The listing builds one solid part. Answer for the finished solid, in the listing's coordinates (mm). A direction names the side the tool comes from. Round coordinates to 2 decimals unless told otherwise and drop trailing zeros. Loops run counter-clockwise (first coordinate to the right, second up) from the corner with the lowest first, then second, coordinate; pieces in that order, holes last. Notation, with made-up numbers: M 24.5,8 L 75.5,8 A20 cw 75.5,46 Z; hole C -11.75,19.25 d5. An arc over 180 degrees is marked long. Put each result on its own line as item: value. Start each with the question number.
(1) Section D-D, the plane z = 0.75 is taken. Count the separate pieces of the cut face and the enclosed holes in it, then the cut area to 3 significant figures.
(2) Which of the six approach directions +Z, -Z, +X, -X, +Y, -Y give full straight-line access (tool end or side, diameter ignored) to faces 4 (the face through (35, 15, 2)), 5 (the face through (37, -2.5, 2)), 6 (the face through (35, -15, 2)), 7 (the face through (-38, -2.5, 2)), 8 (the face through (-5.9, 0, 2))?
(3) Section A-A, the plane x = 4 is taken. Determine the outline of the cut face in (y, z).
(4) Section C-C, the plane x = -8.4 is taken. Determine the outline of the cut face in (y, z), then the cut area to 3 significant figures.
(5) Straight lines are drawn through the part: line 1 (X direction, y = 0, z = 2.15); line 2 (Y direction, x = 11.5, z = 3.95); line 3 (Y direction, x = -8.4, z = 2.6). For each, find the intervals that lie inside material, in ascending order.
(6) Section B-B, the plane y = 0 is taken. Determine the outline of the cut face in (x, z), then the cut area to 3 significant figures.
(7) Determine the mould class of faces 1 (the face through (-35, -15, 2)), 2 (the face through (-25.418, 3.685, 2.465)), 3 (the face through (37, 2.5, 2)) for opening direction X: released by +X, released by -X, zero draft, split by the parting line, or undercut.
(8) Flat-ended cylindrical pins translate along their axes: P1, Ø1.6, axis at x = 18.8, y = 0, coming from the -Z side; P2, Ø1.5, axis at y = -15.5, z = 3, coming from the -X side; P3, Ø2.5, axis at y = 15.5, z = 2.5, coming from the +X side. Find the tip coordinate at first contact, or state that the pin passes through.
```python
from build123d import *

# Parameters (mm, degrees)
ESQUISSE1_W                = 80
ESQUISSE1_H                = 35
BOSS_EXTRU_1_DEPTH         = 5
ESQUISSE3_W                = 5
ESQUISSE3_H                = 5
ENL_V_MAT_EXTRU_1_DEPTH    = 10
R_P_TITION_LIN_AIRE1_COUNT = 4
R_P_TITION_LIN_AIRE1_PITCH = 10
ESQUISSE4_W                = 5
ESQUISSE4_H                = 5
ENL_V_MAT_EXTRU_2_DEPTH    = 10
R_P_TITION_LIN_AIRE2_COUNT = 4
R_P_TITION_LIN_AIRE2_PITCH = 10
ESQUISSE6_W                = 22.2
ESQUISSE6_H                = 11.8
ENL_V_MAT_EXTRU_5_DEPTH    = 10
ESQUISSE7_R                = 1
ESQUISSE7_R_2              = 0.999214349
ENL_V_MAT_EXTRU_7_DEPTH    = 10
ESQUISSE8_R                = 4.5
ENL_V_MAT_EXTRU_8_DEPTH    = 10
ENL_V_MAT_EXTRU_9_DEPTH    = 10


with BuildPart() as part:
    # Esquisse1 → Boss.-Extru.1 (new body)
    with BuildSketch(Plane.XY):
        Rectangle(ESQUISSE1_W, ESQUISSE1_H)
    extrude(amount=BOSS_EXTRU_1_DEPTH)

    # Esquisse3 → Enlèv. mat.-Extru.1 (cut)
    with BuildSketch(Plane.XY):
        with Locations((37.5, -15)):
            Rectangle(ESQUISSE3_W, ESQUISSE3_H)
    enl_v_mat_extru_1 = extrude(amount=ENL_V_MAT_EXTRU_1_DEPTH, mode=Mode.SUBTRACT)

    # Répétition linéaire1: Enlèv. mat.-Extru.1 ×4
    with Locations(*[(0, i * R_P_TITION_LIN_AIRE1_PITCH, 0) for i in range(1, R_P_TITION_LIN_AIRE1_COUNT)]):
        add(enl_v_mat_extru_1, mode=Mode.SUBTRACT)

    # Esquisse4 → Enlèv. mat.-Extru.2 (cut)
    with BuildSketch(Plane.XY):
        with Locations((-37.5, -15)):
            Rectangle(ESQUISSE4_W, ESQUISSE4_H)
    enl_v_mat_extru_2 = extrude(amount=ENL_V_MAT_EXTRU_2_DEPTH, mode=Mode.SUBTRACT)

    # Répétition linéaire2: Enlèv. mat.-Extru.2 ×4
    with Locations(*[(0, i * R_P_TITION_LIN_AIRE2_PITCH, 0) for i in range(1, R_P_TITION_LIN_AIRE2_COUNT)]):
        add(enl_v_mat_extru_2, mode=Mode.SUBTRACT)

    # Esquisse6 → Enlèv. mat.-Extru.5 (cut)
    with BuildSketch(Plane.XY):
        with Locations((5.2, 0)):
            Rectangle(ESQUISSE6_W, ESQUISSE6_H)
    extrude(amount=ENL_V_MAT_EXTRU_5_DEPTH, mode=Mode.SUBTRACT)

    # Esquisse7 → Enlèv. mat.-Extru.7 (cut)
    with BuildSketch(Plane.XY):
        with Locations((18.8, 0)):
            Circle(ESQUISSE7_R)
        with Locations((-8.4, 0)):
            Circle(ESQUISSE7_R_2)
    extrude(amount=ENL_V_MAT_EXTRU_7_DEPTH, mode=Mode.SUBTRACT)

    # Esquisse8 → Enlèv. mat.-Extru.8 (cut)
    with BuildSketch(Plane(origin=(0, 0, 0), x_dir=(-1, 0, 0), z_dir=(0, 0, -1))):
        with Locations((28, 0)):
            Circle(ESQUISSE8_R)
    enl_v_mat_extru_8 = extrude(amount=-ENL_V_MAT_EXTRU_8_DEPTH, mode=Mode.SUBTRACT)

    # Esquisse9 → Enlèv. mat.-Extru.9 (cut)
    with BuildSketch(Plane(origin=(0, 0, 0), x_dir=(-1, 0, 0), z_dir=(0, 0, -1))):
        Polygon((32.25, -1.479019946), (35, -2.5), (35, -7.5), (28.260126937, -4.492475262), align=None)
    enl_v_mat_extru_9 = extrude(amount=-ENL_V_MAT_EXTRU_9_DEPTH, mode=Mode.SUBTRACT)

    # Symétrie1: Enlèv. mat.-Extru.8, Enlèv. mat.-Extru.9 across plane
    add(enl_v_mat_extru_8.mirror(Plane(origin=(0, 0, 0), x_dir=(0, 0, 1), z_dir=(1, 0, 0))), mode=Mode.SUBTRACT)
    add(enl_v_mat_extru_9.mirror(Plane(origin=(0, 0, 0), x_dir=(0, 0, 1), z_dir=(1, 0, 0))), mode=Mode.SUBTRACT)


solid = part.part
```
Recorded:
1. separate pieces: 1
1. enclosed holes: 3
1. area: 2,160 mm²
2. face 4: +Z, -Z, +X, +Y
2. face 5: +Z, -Z, +X
2. face 6: +Z, -Z, +X, -Y
2. face 7: +Z, -Z, -X
2. face 8: +Z, -Z
3. outline: M -17.5,0 L -5.9,0 L -5.9,5 L -17.5,5 Z; M 5.9,0 L 17.5,0 L 17.5,5 L 5.9,5 Z
4. outline: M -17.5,0 L -1,0 L -1,5 L -17.5,5 Z; M 1,0 L 17.5,0 L 17.5,5 L 1,5 Z
4. area: 165 mm²
5. line 1: x = -40 to -32.5, -23.5 to -9.4, -7.4 to -5.9, 16.3 to 17.8, 19.8 to 23.5, 32.5 to 40
5. line 2: y = -17.5 to -5.9, 5.9 to 17.5
5. line 3: y = -17.5 to -1, 1 to 17.5
6. outline: M -40,0 L -32.5,0 L -32.5,5 L -40,5 Z; M -23.5,0 L -9.4,0 L -9.4,5 L -23.5,5 Z; M -7.4,0 L -5.9,0 L -5.9,5 L -7.4,5 Z; M 16.3,0 L 17.8,0 L 17.8,5 L 16.3,5 Z; M 19.8,0 L 23.5,0 L 23.5,5 L 19.8,5 Z; M 32.5,0 L 40,0 L 40,5 L 32.5,5 Z
6. area: 179 mm²
7. face 1: released by -X
7. face 2: undercut
7. face 3: zero draft
8. P1: passes through
8. P2: stops at x = -35
8. P3: stops at x = 35
